The model under review builds one solid part; all positions refer to its coordinate system, in mm. Face numbers are marked on the shaded views. Round coordinates to 2 decimals unless told otherwise and drop trailing zeros. Loops run counter-clockwise (first coordinate to the right, second up) from the corner with the lowest first, then second, coordinate; pieces in that order, holes last. Notation, with made-up numbers: (-24, 14.5) -> (-19, 14.5) arc R37 ccw to (-19, 52.5) -> close; hole circle Ø2 at (84.25, 58.5). An arc over 180 degrees is marked (long way). Write each question's results on one line, items separated by ' | '. Start each with the question number.
Item 1: We need section B-B (x = 16). Give the boundary of the cut face in (y, z) (3 decimals), and give its area (3 significant figures).
Item 2: For L1, parallel to Y at x = 0, z = -89; L2, parallel to Y at x = 0, z = 97; L3, parallel to Z at x = -26, y = 5 (3 decimals), list the stretches that pass through material, from the lowest coordinate up. Write a range as from..to.
Item 3: We need section D-D (z = -87.5). Give the boundary of the cut face in (x, y) (1 decimal).
Item 4: We need section C-C (x = 5.5). Give the boundary of the cut face in (y, z) (3 decimals).
Item 5: We need section A-A (y = -7). Give the boundary of the cut face in (x, z) (3 decimals), and give its area (3 significant figures).
Item 6: Clearance check with flat-ended pins moving along their axes: pin 1 Ø1 at (x, z) = (25.5, 47) entering from +Y; pin 2 Ø3 at (x, y) = (-30.96, 0) entering from +Z; pin 3 Ø4 at (x, y) = (0, -30.96) entering from -Z. State where each tip first meets the part, or that it passes through.
Item 7: Mouldability with a two-part tool opening along Y and no side actions: class the marked faces 1, 2 and 3 as pulls with the +Y half, pulls with the -Y half, needs draft (parallel to the pull), parting line crosses it, or undercut.
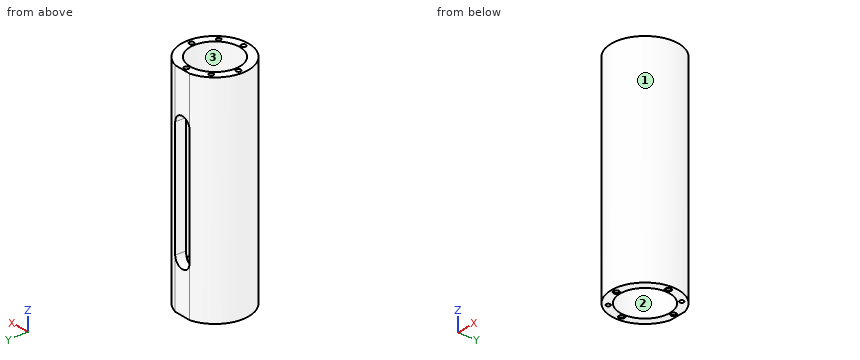
from build123d import *

# Parameters (mm, degrees)
BOLT_CIRCLE_R                      = 36.5125
BOLT_CIRCLE_R_2                    = 25.4
BASE_SHAPE_DEPTH                   = 117.475
BOLT_PATTERN_COUNT                 = 4
SLOT_DEPTH                         = 129.3226439
SKETCH17_R                         = 26.924
INNER_STEP_DEPTH                   = 38.1
EXTRUDE1_DEPTH                     = 129.322644049
EXTRUDE1_DEPTH_BACK                = 129.322644049
SKETCH20_W                         = 37.44274537
SKETCH20_H                         = 1.704436823
ALIGNMENT_PIN_HOLES_D              = 4.7625
ALIGNMENT_PIN_HOLES_DEPTH          = 12.7
ALIGNMENT_PIN_HOLES_TIP            = 1.430799349
F_3_16_0_1875_DIAMETER_HOLE1_D     = 4.7625
F_3_16_0_1875_DIAMETER_HOLE1_DEPTH = 12.7
F_3_16_0_1875_DIAMETER_HOLE1_TIP   = 1.430799349


with BuildPart() as part:
    # Bolt circle → Base shape (new, symmetric)
    with BuildSketch(Plane.XY):
        Circle(BOLT_CIRCLE_R)
        Circle(BOLT_CIRCLE_R_2, mode=Mode.SUBTRACT)
    extrude(amount=BASE_SHAPE_DEPTH, both=True)

    # Sketch10 → Hole Wizard 1_4-20 _1 (revolve, cut)
    with BuildSketch(Plane(origin=(0, 30.95625, -117.475), x_dir=(0, 1, 0), z_dir=(1, 0, 0))):
        Polygon((0, 0), (0, 20.583816902), (2.5527, 19.05), (2.5527, 0.6223), (3.175, 0), align=None)
    hole_wizard_1_4_20_1 = revolve(axis=Axis((0, 30.95625, -123.825), (0, 0, 1)), mode=Mode.SUBTRACT)

    # Sketch11 → Hole Wizard 1_4-20 _2 (revolve, cut)
    with BuildSketch(Plane(origin=(0, 30.95625, 117.475), x_dir=(0, -1, 0), z_dir=(1, 0, 0))):
        Polygon((0, 0), (0, 20.583816902), (2.5527, 19.05), (2.5527, 0), align=None)
    hole_wizard_1_4_20_2 = revolve(axis=Axis((0, 30.95625, 123.825), (0, 0, -1)), mode=Mode.SUBTRACT)

    # Bolt pattern: Hole Wizard 1_4-20 _1, Hole Wizard 1_4-20 _2 ×4 about axis
    bolt_pattern_axis = Axis((0, 0, 0), (0, 0, 1))
    add([hole_wizard_1_4_20_1.rotate(bolt_pattern_axis, i * 360 / BOLT_PATTERN_COUNT) for i in range(1, BOLT_PATTERN_COUNT)], mode=Mode.SUBTRACT)
    add([hole_wizard_1_4_20_2.rotate(bolt_pattern_axis, i * 360 / BOLT_PATTERN_COUNT) for i in range(1, BOLT_PATTERN_COUNT)], mode=Mode.SUBTRACT)

    # Sketch14 → Slot (cut, through all)
    with BuildSketch(Plane(origin=(0, 0, 0), x_dir=(1, 0, 0), z_dir=(0, 1, 0))):
        with BuildLine():
            Line((-9.525, 63.5), (-9.525, -63.5))
            ThreePointArc((-9.525, -63.5), (0, -73.025), (9.525, -63.5))
            Line((9.525, -63.5), (9.525, 63.5))
            ThreePointArc((9.525, 63.5), (0, 73.025), (-9.525, 63.5))
        make_face()
    extrude(amount=SLOT_DEPTH, mode=Mode.SUBTRACT)

    # Sketch17 → Inner Step (cut)
    with BuildSketch(Plane.XY.offset(117.475)):
        Circle(SKETCH17_R)
    inner_step = extrude(amount=-INNER_STEP_DEPTH, mode=Mode.SUBTRACT)

    # Step Mirror: Inner Step across plane
    add(inner_step.mirror(Plane.XY), mode=Mode.SUBTRACT)

    # Sketch20 → Extrude1 (cut, two sides: drawn at the far end of the back side and taken through both)
    with BuildSketch(Plane.XY.offset(-EXTRUDE1_DEPTH_BACK)):
        with Locations((-0.049008829, 36.100438668)):
            Rectangle(SKETCH20_W, SKETCH20_H)
    extrude(amount=EXTRUDE1_DEPTH + EXTRUDE1_DEPTH_BACK, mode=Mode.SUBTRACT)

    # Alignment_pin_holes
    with Locations(Plane.XY.offset(117.475)):
        with Locations((-21.889374295, 21.889374295), (21.889374295, -21.889374295)):
            Hole(ALIGNMENT_PIN_HOLES_D / 2, depth=ALIGNMENT_PIN_HOLES_DEPTH)
            with Locations((0, 0, -(ALIGNMENT_PIN_HOLES_DEPTH + ALIGNMENT_PIN_HOLES_TIP / 2))):  # 118° drill point
                Cone(0, ALIGNMENT_PIN_HOLES_D / 2, ALIGNMENT_PIN_HOLES_TIP, mode=Mode.SUBTRACT)

    # 3_16 _0.1875_ Diameter Hole1
    with Locations(Plane(origin=(0, 0, -117.475), x_dir=(-1, 0, 0), z_dir=(0, 0, -1))):
        with Locations((-21.889374295, 21.889374295), (21.889374295, -21.889374295)):
            Hole(F_3_16_0_1875_DIAMETER_HOLE1_D / 2, depth=F_3_16_0_1875_DIAMETER_HOLE1_DEPTH)
            with Locations((0, 0, -(F_3_16_0_1875_DIAMETER_HOLE1_DEPTH + F_3_16_0_1875_DIAMETER_HOLE1_TIP / 2))):  # 118° drill point
                Cone(0, F_3_16_0_1875_DIAMETER_HOLE1_D / 2, F_3_16_0_1875_DIAMETER_HOLE1_TIP, mode=Mode.SUBTRACT)


solid = part.part
Here are the results:
1) outline: (-32.82, -117.475) -> (-21.654, -117.475) -> (-21.654, -79.375) -> (-19.727, -79.375) -> (-19.727, 79.375) -> (-21.654, 79.375) -> (-21.654, 117.475) -> (-32.82, 117.475) -> close; (19.727, -79.375) -> (21.654, -79.375) -> (21.654, -117.475) -> (32.82, -117.475) -> (32.82, 117.475) -> (21.654, 117.475) -> (21.654, 79.375) -> (19.727, 79.375) -> close | area: 5,860 mm2
2) L1: y = -36.51..-26.92, 26.92..35.25 | L2: y = -36.51..-31.14, -30.78..-26.92, 26.92..30.78, 31.14..35.25 | L3: z = -79.375..79.375
3) outline: (-9.5, 35.2) arc R36.5 ccw (long way) to (9.5, 35.2) -> close; hole circle Ø53.8 at (0, 0)
4) outline: (-36.096, -117.475) -> (-26.356, -117.475) -> (-26.356, -79.375) -> (-24.797, -79.375) -> (-24.797, 79.375) -> (-26.356, 79.375) -> (-26.356, 117.475) -> (-36.096, 117.475) -> close; (24.797, -79.375) -> (26.356, -79.375) -> (26.356, -117.475) -> (35.248, -117.475) -> (35.248, -71.277) -> (24.797, -71.277) -> close; (24.797, 71.277) -> (35.248, 71.277) -> (35.248, 117.475) -> (26.356, 117.475) -> (26.356, 79.375) -> (24.797, 79.375) -> close
5) outline: (-35.835, -117.475) -> (-25.998, -117.475) -> (-25.998, -79.375) -> (-24.416, -79.375) -> (-24.416, 79.375) -> (-25.998, 79.375) -> (-25.998, 117.475) -> (-35.835, 117.475) -> close; (24.416, -79.375) -> (25.998, -79.375) -> (25.998, -117.475) -> (35.835, -117.475) -> (35.835, 117.475) -> (25.998, 117.475) -> (25.998, 79.375) -> (24.416, 79.375) -> close | area: 5,120 mm2
6) pin 1: stops at y = 26.61 | pin 2: stops at z = 97.79 | pin 3: stops at z = -98.1
7) face 1: parting line crosses it | face 2: undercut | face 3: undercut
